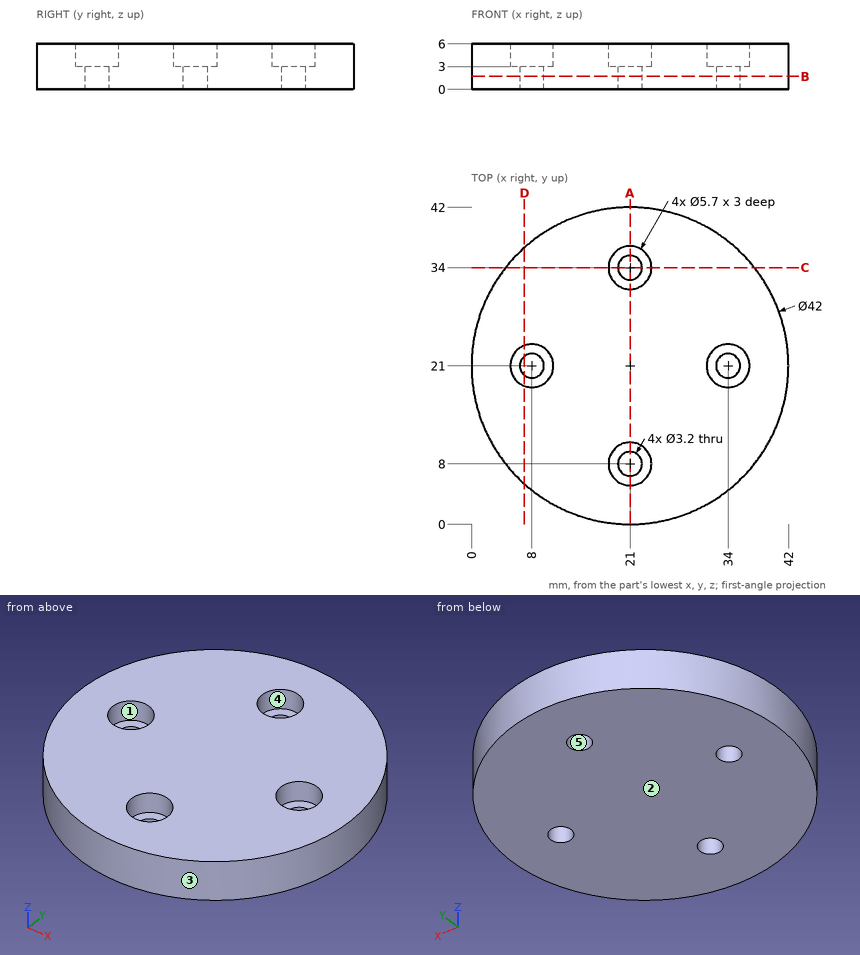
Source: three-view drawing plus pictorial views. Frame: mm from the lowest corner of the part. A direction names the side the tool comes from. Coordinates: 2 decimals unless noted, no trailing zeros. Loops run counter-clockwise (first coordinate to the right, second up) from the corner with the lowest first, then second, coordinate; pieces in that order, holes last. Notation, with made-up numbers: (-21, 31) - (30, 31) arc R25 ccw to (30, 62) - close; hole circle Ø9 at (-36, 9). An arc over 180 degrees is marked (long way). One line per item, written item: value. Start each with the question number.
1. Section C-C (y = 34). Return the cut outline in (x, z).
2. Set-up query: the marked faces 4 and 5. Return all of +Z, -Z, +X, -X, +Y, -Y with unobstructed straight access to the full face (end or side cutting, diameter ignored); none if empty.
3. Contact query for flat-ended pins moving along their axis: P1, Ø1.5, axis at y = 30.5, z = 4, coming from the +X side; P2, Ø3, axis at x = 7.5, y = 20.5, coming from the +Z side; P3, Ø3, axis at x = 28.5, z = 2.5, coming from the -Y side. Output: stop coordinate, or through.
4. Section D-D (x = 7). Return the cut outline in (y, z), and give its area (3 significant figures).
5. Ray query, L1, parallel to Y at x = 21, z = 5.3; L2, parallel to Z at x = 36.5, y = 20.5; L3, parallel to X at y = 33, z = 4.15. Return the intervals inside material, ascending.
6. Section B-B (z = 1.7). Return the cut outline in (x, y).
7. Section A-A (x = 21). Return the cut outline in (y, z).
8. Mould query, pull axis X, two halves, no side actions, for the marked faces 1, 2 and 3. Classes: pulls with the +X half, pulls with the -X half, needs draft (parallel to the pull), parting line crosses it, or undercut.
Verdict:
1. outline: (4.51, 0) - (19.4, 0) - (19.4, 3) - (18.15, 3) - (18.15, 6) - (4.51, 6) - close; (22.6, 0) - (37.49, 0) - (37.49, 6) - (23.85, 6) - (23.85, 3) - (22.6, 3) - close
2. face 4: +Z
2. face 5: +Z, -Z
3. P1: stops at x = 40.09
3. P2: stops at z = 3
3. P3: stops at y = 0.88
4. outline: (5.35, 0) - (19.75, 0) - (19.75, 3) - (18.33, 3) - (18.33, 6) - (5.35, 6) - close; (22.25, 0) - (36.65, 0) - (36.65, 6) - (23.67, 6) - (23.67, 3) - (22.25, 3) - close
4. area: 164 mm2
5. L1: y = 0 to 5.15, 10.85 to 31.15, 36.85 to 42
5. L2: z = 0 to 3
5. L3: x = 3.77 to 18.33, 23.67 to 38.23
6. outline: circle Ø42 at (21, 21); hole circle Ø3.2 at (8, 21); hole circle Ø3.2 at (21, 8); hole circle Ø3.2 at (21, 34); hole circle Ø3.2 at (34, 21)
7. outline: (0, 0) - (6.4, 0) - (6.4, 3) - (5.15, 3) - (5.15, 6) - (0, 6) - close; (9.6, 0) - (32.4, 0) - (32.4, 3) - (31.15, 3) - (31.15, 6) - (10.85, 6) - (10.85, 3) - (9.6, 3) - close; (35.6, 0) - (42, 0) - (42, 6) - (36.85, 6) - (36.85, 3) - (35.6, 3) - close
8. face 1: undercut
8. face 2: needs draft
8. face 3: parting line crosses it
